Build history of the part. All positions in model axes, mm. A direction names the side the tool comes from. Round coordinates to 2 decimals unless told otherwise and drop trailing zeros. Write each loop counter-clockwise with the first axis right and the second up, starting at its lowest first coordinate (ties: lowest second). Pieces come first, ordered by that corner, then holes. Notation, with made-up numbers: (57.25, -2) - (84.25, -2) arc R27 ccw to (84.25, 26) - close; hole circle Ø11 at (86.5, 43.25). An arc over 180 degrees is marked (long way). Answer as a JSON object with one key per item and string values. Group by question number.
Item 1: Which spindle directions (+Z, -Z, +X, -X, +Y, -Y) get a long thin tool onto all of the face, cutting with end or side? Do faces 5 (the flat face through (14.877, 276.362, 1168.726)), 6 (the flat face through (14.88, 201.72, 1213.45)). Say none if no direction does.
Item 2: Flat gauge pins, fed straight in: pin 1 (5 mm diameter, centred on y = 144.9, z = 1245.97, fed in from +X); pin 2 (2 mm diameter, centred on x = 14.5, y = 225, fed in from +Z). Where does each tip first touch, or does it go through?
Item 3: Slice it at B-B, the plane z = 1154.5. List the corners of the cut face in (x, y) (3 decimals).
Item 4: Slice it at D-D, the plane z = 1213.5. List the corners of the cut face in (x, y), then the cut area to 3 significant figures.
Item 5: Probe line 1 (Z direction, x = 13.65, y = 145); line 2 (Y direction, x = 15.7, z = 1159); line 3 (Y direction, x = 13.35, z = 1153). List the from-to ranges inside material, lowest first. Write a range as from..to.
Item 6: Slice it at C-C, the plane y = 161. List the corners of the cut face in (x, z), then the cut area to 3 significant figures.
Item 7: Slice it at A-A, the plane x = 13.65. Give the number of separate pieces and of enclosed holes in the cut face, then the cut area to 3 significant figures.
Item 8: Two-plate mould, pull along Y, no slides. Class faces 1 (the cylindrical face through (14.88, 342.55, 1133.2)), 2 (the cylindrical face through (14.877, 140.875, 1254.605)), 3 (the cylindrical face through (14.943, 253.16, 1173.375)), 4 (the flat face through (12.529, 222, 1180)): +Y half, -Y half, draft (parallel to the pull), parting line (faces both ways), or undercut.
from build123d import *

# Parameters (mm, degrees)
BOSS_EXTRUDE1_START = 12.528612
SKETCH2_R           = 3.175
SKETCH2_R_2         = 5.781305793
SKETCH2_R_3         = 6.382098514
BOSS_EXTRUDE1_DEPTH = 4.7625
FILLET1_R           = 9.525


with BuildPart() as part:
    # Sketch2 → Boss-Extrude1 (new body)
    with BuildSketch(Plane(origin=(0, 0, 0), x_dir=(0, 0, -1), z_dir=(1, 0, 0)).offset(BOSS_EXTRUDE1_START)):
        with BuildLine():
            ThreePointArc((-1144.374252892, 135.379574554), (-1135.977897239, 140.407148985), (-1136.445227254, 150.182469725))
            Line((-1136.445227254, 150.182469725), (-1164.81319381, 192.799900886))
            Line((-1164.81319381, 192.799900886), (-1112.182497939, 318.610437742))
            Line((-1112.182497939, 318.610437742), (-1095.74378362, 357.906203065))
            Line((-1095.74378362, 357.906203065), (-1137.77556383, 350.998384801))
            Line((-1137.77556383, 350.998384801), (-1162.839331646, 346.879217061))
            ThreePointArc((-1162.839331646, 346.879217061), (-1169.029486958, 343.038885374), (-1170.695468345, 335.947293432))
            Line((-1170.695468345, 335.947293432), (-1164.57634177, 298.423200658))
            Line((-1164.57634177, 298.423200658), (-1173.106250375, 253.07288466))
            Line((-1173.106250375, 253.07288466), (-1253.464218567, 150.788964003))
            ThreePointArc((-1253.464218567, 150.788964003), (-1254.540886843, 140.740633182), (-1245.974252892, 135.379574554))
            Line((-1245.974252892, 135.379574554), (-1144.374252892, 135.379574554))
        make_face()
        with Locations((-1245.974252892, 144.904574554)):
            Circle(SKETCH2_R, mode=Mode.SUBTRACT)
        with Locations((-1220.574252892, 144.904574554)):
            Circle(SKETCH2_R, mode=Mode.SUBTRACT)
        with Locations((-1185.371762566, 168.336842549)):
            Circle(SKETCH2_R, mode=Mode.SUBTRACT)
        with Locations((-1169.774252892, 144.904574554)):
            Circle(SKETCH2_R, mode=Mode.SUBTRACT)
        with Locations((-1144.374252892, 144.904574554)):
            Circle(SKETCH2_R, mode=Mode.SUBTRACT)
        with Locations((-1175.56927224, 191.769110545)):
            Circle(SKETCH2_R, mode=Mode.SUBTRACT)
        with Locations((-1164.176264161, 249.021430388)):
            Circle(SKETCH2_R_2, mode=Mode.SUBTRACT)
        with Locations((-1144.465794272, 266.120118002)):
            Circle(SKETCH2_R, mode=Mode.SUBTRACT)
        with Locations((-1154.90639106, 298.305859313)):
            Circle(SKETCH2_R_3, mode=Mode.SUBTRACT)
        with Locations((-1130.772088763, 298.854103619)):
            Circle(SKETCH2_R, mode=Mode.SUBTRACT)
        with Locations((-1161.294643743, 337.48030413)):
            Circle(SKETCH2_R, mode=Mode.SUBTRACT)
        with Locations((-1136.230875927, 341.59947187)):
            Circle(SKETCH2_R, mode=Mode.SUBTRACT)
        with Locations((-1120.969598437, 322.286371614)):
            Circle(SKETCH2_R, mode=Mode.SUBTRACT)
    extrude(amount=BOSS_EXTRUDE1_DEPTH)

    # Fillet1
    fillet1_edges = [part.edges().sort_by_distance(p)[0] for p in [
        (14.909862, 357.906203065, 1095.74378362),
        (14.909862, 192.799900886, 1164.81319381),
        (14.909862, 253.07288466, 1173.106250375),
        (14.909862, 298.423200658, 1164.57634177),
    ]]
    fillet(fillet1_edges, radius=FILLET1_R)


solid = part.part
Geometry says:
{
 "1": {"face 5": "+Z, +X, -X", "face 6": "+Z, +X, -X, +Y"},
 "2": {"pin 1": "passes through", "pin 2": "stops at z = 1195.95"},
 "3": {"outline": "(12.529, 135.38) - (17.291, 135.38) - (17.291, 177.306) - (12.529, 177.306) - close; (12.529, 217.453) - (17.291, 217.453) - (17.291, 291.937) - (12.529, 291.937) - close; (12.529, 304.675) - (17.291, 304.675) - (17.291, 348.25) - (12.529, 348.25) - close"},
 "4": {"outline": "(12.53, 135.38) - (17.29, 135.38) - (17.29, 201.66) - (12.53, 201.66) - close", "area": "316 mm^2"},
 "5": {"line 1": "z = 1134.85..1141.2, 1147.55..1166.6, 1172.95..1217.4, 1223.75..1242.8, 1249.15..1255.5", "line 2": "y = 135.38..184.07, 206.7..246.45, 251.6..293.41, 303.2..335.29, 339.67..347.51", "line 3": "y = 135.38..175.05, 221.04..292.22, 304.4..348.5"},
 "6": {"outline": "(12.53, 1143.65) - (17.29, 1143.65) - (17.29, 1245.44) - (12.53, 1245.44) - close", "area": "485 mm^2"},
 "7": {"separate pieces": "1", "enclosed holes": "13", "area": "12,400 mm^2"},
 "8": {"face 1": "undercut", "face 2": "parting line", "face 3": "+Y half", "face 4": "draft"}
}
